Study the drawing (mm; zero at the part's minimum x, y, z) and answer. A direction names the side the tool comes from. Coordinates: 2 decimals unless noted, no trailing zeros. Order: outer loops, then holes, each group sorted by start corner. A loop starts at its lowest first (then second) coordinate and runs counter-clockwise, first axis right, second up. Notation, with made-up numbers: (33.5, 60) -> (67.5, 60) arc R24 ccw to (67.5, 77) -> close; hole circle Ø5 at (50, -1.75). An arc over 180 degrees is marked (long way). Answer as CSV lines item,"result". Start each with the question number.
Item 1: Each of these flat-tipped pins is pushed along its axis until it touches: pin 1 Ø0.9 at (x, y) = (4, 4.5) entering from +Z; pin 2 Ø1.5 at (x, z) = (1, 21.5) entering from +Y; pin 3 Ø2 at (y, z) = (6.5, 6) entering from +X. Where does it stop, or does it pass through?
Item 2: For a pull along X with two mould halves and no side action, classify the marked faces 3, 4 and 5 as pulls with the +X half, pulls with the -X half, needs draft (parallel to the pull), parting line crosses it, or undercut.
Item 3: Section D-D (z = 11) is taken. Write down the section's boundary in (x, y).
Item 4: Straight lines are drawn through the part: L1, parallel to Y at x = 4, z = 21.65; L2, parallel to Z at x = 3.75, y = 3.25; L3, parallel to Y at x = 2, z = 10. For each, find the intervals that lie inside material, in ascending order.
Item 5: Which of the six approach directions +Z, -Z, +X, -X, +Y, -Y give full straight-line access (tool end or side, diameter ignored) to the marked faces 1 and 2?
Item 6: Section A-A (y = 4) is taken. Write down the section's boundary in (x, z).
Item 7: Section B-B (z = 2) is taken. Write down the section's boundary in (x, y), then the cut area to 3 significant figures.
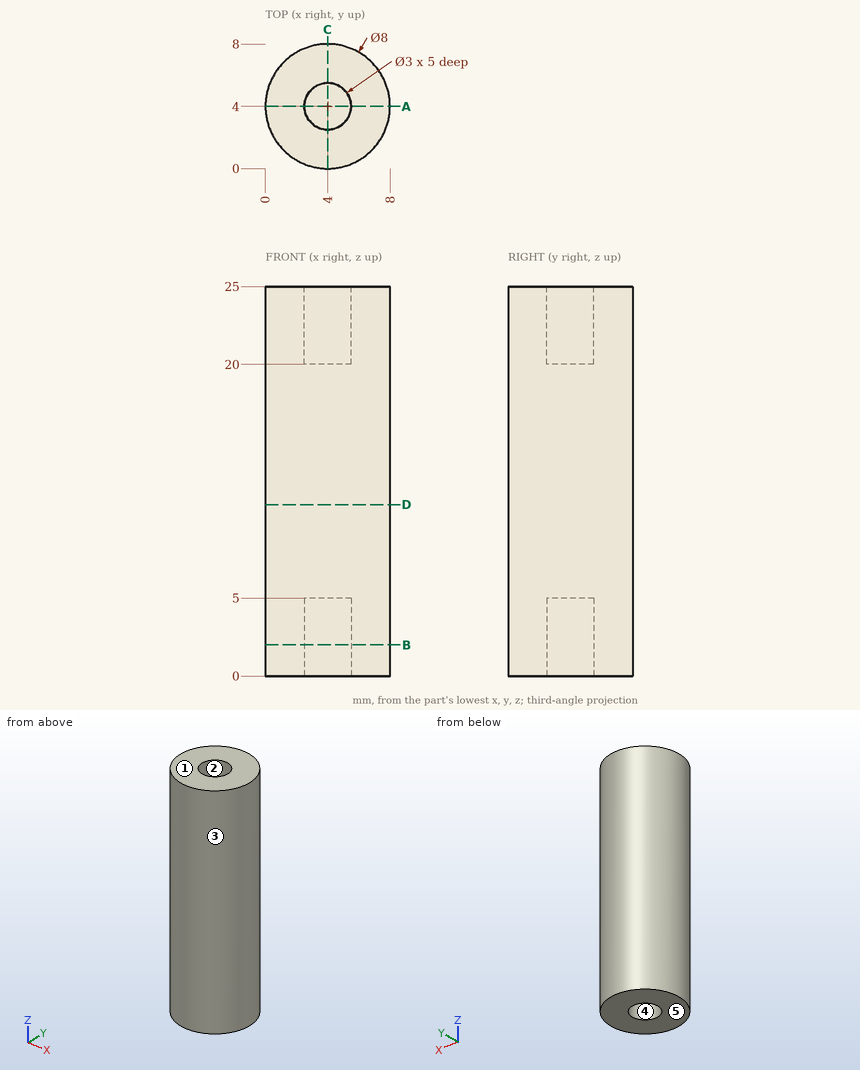
Checked values:
1,pin 1,"stops at z = 20"
1,pin 2,"stops at y = 7.31"
1,pin 3,"stops at x = 7.71"
2,face 3,"parting line crosses it"
2,face 4,"undercut"
2,face 5,"needs draft"
3,outline,"circle Ø8 at (4, 4)"
4,L1,"y = 0 to 2.5, 5.5 to 8"
4,L2,"z = 5 to 20"
4,L3,"y = 0.54 to 7.46"
5,face 1,"+Z, +X, -X, +Y, -Y"
5,face 2,"+Z"
6,outline,"(0, 0) -> (2.5, 0) -> (2.5, 5) -> (5.5, 5) -> (5.5, 0) -> (8, 0) -> (8, 25) -> (5.5, 25) -> (5.5, 20) -> (2.5, 20) -> (2.5, 25) -> (0, 25) -> close"
7,outline,"circle Ø8 at (4, 4); hole circle Ø3 at (4, 4)"
7,area,"43.2 mm^2"
